Design review of the part built by this model. Coordinates are the model's own, in mm. Coordinates: 2 decimals unless noted, no trailing zeros. Write each loop counter-clockwise with the first axis right and the second up, starting at its lowest first coordinate (ties: lowest second). Pieces come first, ordered by that corner, then holes. Notation, with made-up numbers: (-34.5, 48.25) -> (-9.5, 48.25) arc R27 cw to (-9.5, 85.25) -> close; hole circle Ø10 at (44.25, 44). An arc over 180 degrees is marked (long way). One line per question, with ' | ' between items. Start each with the question number.
Q1. Add section B-B on y = 84.5. State the section outline as (x, z) points.
Q2. Add section A-A on z = 3.2. State the section outline as (x, y) points, and give its area (3 significant figures).
Q3. Draft analysis for pull direction X (two halves, no side actions). For faces 1 (the cylindrical face through (-3, 0, 3)), 2 (the cylindrical face through (-0.546, 69.02, 0.051)), 3 (the flat face through (-1, -3, 0)), state which applies: pulls with the +X half, pulls with the -X half, needs draft (parallel to the pull), parting line crosses it, or undercut.
Q4. For P1, Ø2, axis at x = -1.5, y = 69.5, coming from the +Z side; P2, Ø3, axis at x = -3, z = 4, coming from the -Y side; P3, Ø2, axis at y = 61.5, z = 1, coming from the -X side, all flat-tipped, find the tip position at first contact; note any pin that passes through.
Q5. Wall thickness on probe 1 along Y at (x, z) = (0, 2.2); probe 2 along X at (y, z) = (0, 2.75); probe 3 along Y at (x, z) = (1, 2.8): over which ranges is each line inside the solid? List them lowest first.
from build123d import *

# Parameters (mm, degrees)
SKETCH_1_R          = 4
EXTRUDE_1_DEPTH     = 5
SKETCH_3_R          = 2.5
EXTRUDE_2_DEPTH     = 140
SKETCH_2_R          = 3
CUT_EXTRUDE_1_DEPTH = 5


with BuildPart() as part:
    # 草图1 → 凸台-拉伸1 (new body)
    with BuildSketch(Plane.XY):
        Circle(SKETCH_1_R)
    extrude(amount=EXTRUDE_1_DEPTH)

    # 草图3 → 凸台-拉伸2 (add)
    with BuildSketch(Plane(origin=(0, 0, 0), x_dir=(1, 0, 0), z_dir=(0, 1, 0))):
        with Locations(Location((0, -2.490986951, 0), (0, 0, 85.133305815))):
            Circle(SKETCH_3_R)
    extrude(amount=EXTRUDE_2_DEPTH)

    # 草图2 → 切除-拉伸1 (cut)
    with BuildSketch(Plane.XY.offset(5)):
        Circle(SKETCH_2_R)
    extrude(amount=-CUT_EXTRUDE_1_DEPTH, mode=Mode.SUBTRACT)


solid = part.part
Output values:
1) outline: circle Ø5 at (0, 2.49)
2) outline: (-2.4, 3.2) arc R4 ccw (long way) to (2.4, 3.2) -> (2.4, 140) -> (-2.4, 140) -> close; hole circle Ø6 at (0, 0) | area: 675 mm2
3) face 1: undercut | face 2: parting line crosses it | face 3: needs draft
4) P1: stops at z = 4.94 | P2: stops at y = -3.71 | P3: stops at x = -2.45
5) probe 1: y = -4 to -3, 3 to 140 | probe 2: x = -4 to -3, 3 to 4 | probe 3: y = -3.87 to -2.83, 2.83 to 140
